```python
from build123d import *

# Parameters (mm, degrees)
BOSS_EXTRUDE1_DEPTH = 6


with BuildPart() as part:
    # Sketch1 → Boss-Extrude1 (new, symmetric)
    with BuildSketch(Plane.XY):
        with BuildLine():
            Line((24.157706093, 16.904121864), (34.157706093, 16.904121864))
            Line((34.157706093, 16.904121864), (34.157706093, -18.095878136))
            Line((34.157706093, -18.095878136), (-25.842293907, -18.095878136))
            Line((-25.842293907, -18.095878136), (-25.842293907, 16.904121864))
            Line((-25.842293907, 16.904121864), (-15.842293907, 16.904121864))
            Line((-15.842293907, 16.904121864), (-15.842293907, 6.904121864))
            Line((-15.842293907, 6.904121864), (-0.842028463, 6.749549236))
            ThreePointArc((-0.842028463, 6.749549236), (4.106185531, 1.698294118), (9.157440649, 6.646508112))
            Line((9.157440649, 6.646508112), (24.157706093, 6.491935484))
            Line((24.157706093, 6.491935484), (24.157706093, 11.07078853))
            Line((24.157706093, 11.07078853), (24.157706093, 16.904121864))
        make_face()
    extrude(amount=BOSS_EXTRUDE1_DEPTH, both=True)


solid = part.part
```
Build history of the part. All positions in model axes, mm. A direction names the side the tool comes from. Round coordinates to 2 decimals unless told otherwise and drop trailing zeros. Write each loop counter-clockwise with the first axis right and the second up, starting at its lowest first coordinate (ties: lowest second). Pieces come first, ordered by that corner, then holes.
1) Band-saw the part on B-B, the plane z = -2.75. List the corners of the cut face in (x, y), and give its area (3 significant figures).
2) Band-saw the part on D-D, the plane x = -3. List the corners of the cut face in (y, z).
3) Band-saw the part on C-C, the plane y = 3.5. List the corners of the cut face in (x, z).
4) Drill centre lines: probe 1 along X at (y, z) = (8, -0.5); probe 2 along X at (y, z) = (6, 0); probe 3 along Y at (x, z) = (-15, -1.5). Where is each one in solid material? Low to high.
5) Mould opens along X. For faces 1 (the flat face through (29, 16.904, 0)), 2 (the flat face through (-25.842, -1, 0)), 3 (the flat face through (-15.842, 12, 0)) say: +X half, -X half, draft (parallel to the pull), parting line (faces both ways), or undercut.
6) 3-axis set-ups, long thin cutter, end or side, ignore diameter. For faces 4 (the flat face through (-21, 16.904, 0)), 5 (the flat face through (24.158, 12, 0)): which of +Z, -Z, +X, -X, +Y, -Y reach the whole face in a straight line?
7) Pin check, flat tip, straight feed: pin 1 (6 mm diameter, centred on x = -11, z = 2.5, fed in from +Y). Stop position of the tip, or through.
8) Band-saw the part on A-A, the plane y = 13. List the corners of the cut face in (x, z).
Ans:
1. outline: (-25.84, -18.1) - (34.16, -18.1) - (34.16, 16.9) - (24.16, 16.9) - (24.16, 6.49) - (9.16, 6.65) arc R5 cw to (-0.84, 6.75) - (-15.84, 6.9) - (-15.84, 16.9) - (-25.84, 16.9) - close
1. area: 1,650 mm2
2. outline: (-18.1, -6) - (6.77, -6) - (6.77, 6) - (-18.1, 6) - close
3. outline: (-25.84, -6) - (0.31, -6) - (0.31, 6) - (-25.84, 6) - close; (8, -6) - (34.16, -6) - (34.16, 6) - (8, 6) - close
4. probe 1: x = -25.84 to -15.84, 24.16 to 34.16
4. probe 2: x = -25.84 to -0.79, 9.11 to 34.16
4. probe 3: y = -18.1 to 6.9
5. face 1: draft
5. face 2: -X half
5. face 3: undercut
6. face 4: +Z, -Z, +X, -X, +Y
6. face 5: +Z, -Z, +Y
7. pin 1: stops at y = 6.89
8. outline: (-25.84, -6) - (-15.84, -6) - (-15.84, 6) - (-25.84, 6) - close; (24.16, -6) - (34.16, -6) - (34.16, 6) - (24.16, 6) - close
